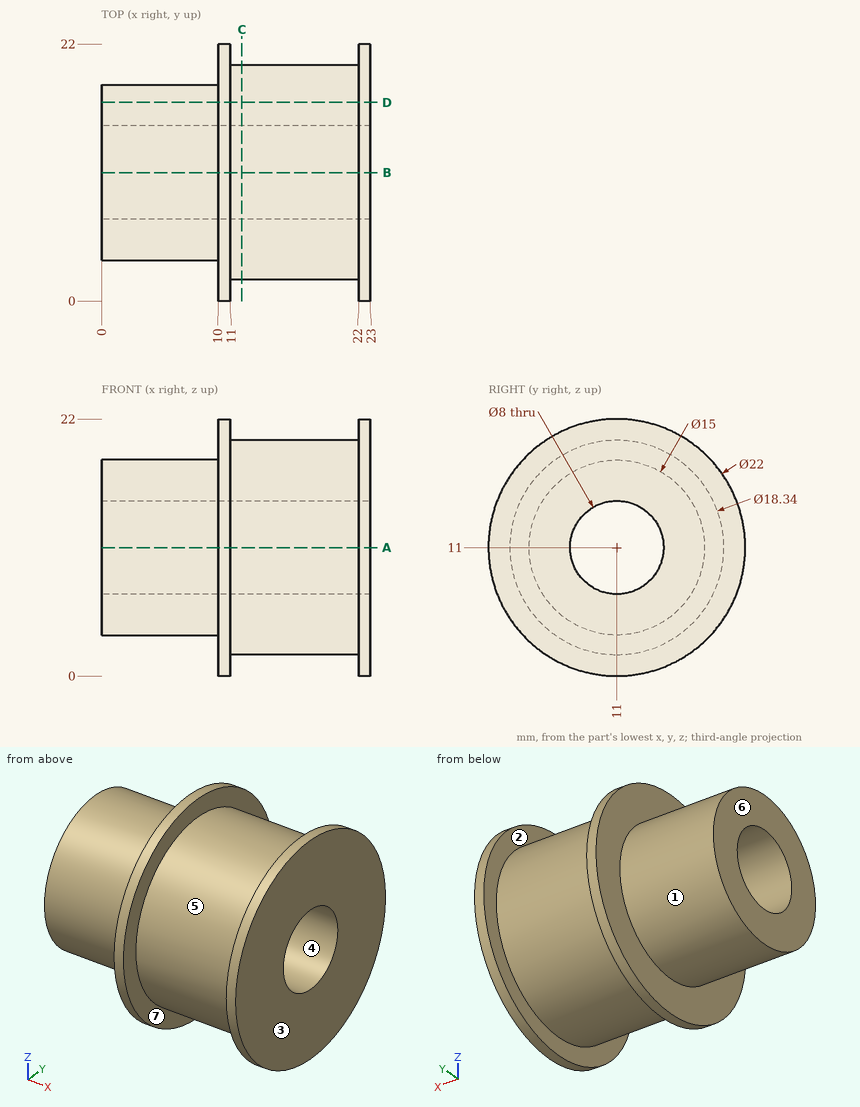
Could you check a few things on this drawing? It's one solid part, dimensions in mm from its lowest x, y, z. A direction names the side the tool comes from. Coordinates: 2 decimals unless noted, no trailing zeros. Loops run counter-clockwise (first coordinate to the right, second up) from the corner with the lowest first, then second, coordinate; pieces in that order, holes last.
1. For the marked faces 1, 2 and 3, which set-ups out of +Z, -Z, +X, -X, +Y, -Y let a thin tool reach every point of the face, with its end or its side?
2. I need wall thicknesses on L1, parallel to Y at x = 7.25, z = 11; L2, parallel to Y at x = 17, z = 11; L3, parallel to X at y = 21.25, z = 7.5. Which ranges of each line are inside material? Lowest first, please.
3. Imagine slicing it at C-C (x = 12). Please give me the cut outline in (y, z).
4. We'd pull the mould along X, two halves only. Please class the marked faces 4, 5, 6 and 7: released by +X, released by -X, zero draft, split by the parting line, or undercut.
5. For P1, Ø8, axis at x = 17.5, y = 15, coming from the -Z side; P2, Ø1, axis at x = 17, y = 4.5, coming from the -Z side; P3, Ø2, axis at x = 15, z = 17.5, coming from the -Y side, each with a flat end and sliding along its axis, tell me the tip position at first contact or that it passes through.
6. Imagine slicing it at A-A (z = 11). Please give me the cut outline in (x, y).
7. Imagine slicing it at D-D (y = 17). Please give me the cut outline in (x, z).
Computed values:
1. face 1: -X
1. face 2: none
1. face 3: +Z, -Z, +X, +Y, -Y
2. L1: y = 3.5 to 7, 15 to 18.5
2. L2: y = 1.83 to 7, 15 to 20.17
2. L3: x = 10 to 11, 22 to 23
3. outline: circle Ø18.34 at (11, 11); hole circle Ø8 at (11, 11)
4. face 4: zero draft
4. face 5: undercut
4. face 6: released by -X
4. face 7: undercut
5. P1: stops at z = 1.83
5. P2: stops at z = 4.07
5. P3: stops at y = 3.66
6. outline: (0, 3.5) - (10, 3.5) - (10, 0) - (11, 0) - (11, 1.83) - (22, 1.83) - (22, 0) - (23, 0) - (23, 7) - (0, 7) - close; (0, 15) - (23, 15) - (23, 22) - (22, 22) - (22, 20.17) - (11, 20.17) - (11, 22) - (10, 22) - (10, 18.5) - (0, 18.5) - close
7. outline: (0, 6.5) - (10, 6.5) - (10, 1.78) - (11, 1.78) - (11, 4.07) - (22, 4.07) - (22, 1.78) - (23, 1.78) - (23, 20.22) - (22, 20.22) - (22, 17.93) - (11, 17.93) - (11, 20.22) - (10, 20.22) - (10, 15.5) - (0, 15.5) - close
